from build123d import *

# Parameters (mm, degrees)
BOSS_EXTRUDE1_DEPTH = 6.35
SKETCH3_R           = 19.685
CUT_EXTRUDE1_DEPTH  = 7.35


with BuildPart() as part:
    # Sketch2 → Boss-Extrude1 (new body)
    with BuildSketch(Plane.XY):
        Polygon((0, 304.8), (0, 12.7), (127, 12.7), (127, 50.8), (254, 50.8), (254, 12.7), (431.8, 12.7), (431.8, 431.8), (215.9, 431.8), align=None)
    extrude(amount=BOSS_EXTRUDE1_DEPTH)

    # Sketch3 → Cut-Extrude1 (cut, through all)
    with BuildSketch(Plane.XY.offset(6.35)):
        with Locations((98.15, 150.3)):
            Circle(SKETCH3_R)
        with Locations((333.65, 150.3)):
            Circle(SKETCH3_R)
    extrude(amount=-CUT_EXTRUDE1_DEPTH, mode=Mode.SUBTRACT)


solid = part.part
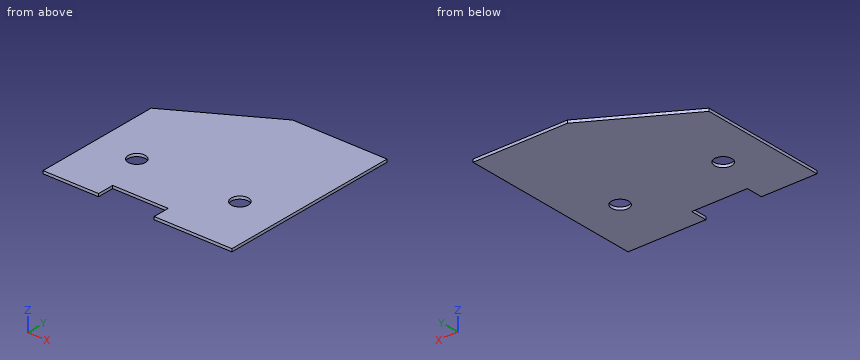
Verification items for the finished model (mm, model axes). Round coordinates to 2 decimals unless told otherwise and drop trailing zeros. Order: outer loops, then holes, each group sorted by start corner. A loop starts at its lowest first (then second) coordinate and runs counter-clockwise, first axis right, second up.
1. Section check D-D on x = 98.15. Record the cut outline in (y, z) (3 decimals).
Final values:
outline: (12.7, 0) - (130.615, 0) - (130.615, 6.35) - (12.7, 6.35) - close; (169.985, 0) - (362.535, 0) - (362.535, 6.35) - (169.985, 6.35) - close
2. Section check A-A on y = 150.3. Record the cut outline in (x, z) (3 decimals), then the cut area to 3 significant figures.
Final values:
outline: (0, 0) - (78.465, 0) - (78.465, 6.35) - (0, 6.35) - close; (117.835, 0) - (313.965, 0) - (313.965, 6.35) - (117.835, 6.35) - close; (353.335, 0) - (431.8, 0) - (431.8, 6.35) - (353.335, 6.35) - close
area: 2,240 mm2
3. Thickness scan on L1, parallel to X at y = 30, z = 6.25; L2, parallel to Y at x = 333.65, z = 3.5 (3 decimals); L3, parallel to Y at x = 238.5, z = 5. Record the ranges inside material, lowest first.
Final values:
L1: x = 0 to 127, 254 to 431.8
L2: y = 12.7 to 130.615, 169.985 to 431.8
L3: y = 50.8 to 431.8
4. Section check B-B on x = 333.65. Record the cut outline in (y, z) (3 decimals), then the cut area to 3 significant figures.
Final values:
outline: (12.7, 0) - (130.615, 0) - (130.615, 6.35) - (12.7, 6.35) - close; (169.985, 0) - (431.8, 0) - (431.8, 6.35) - (169.985, 6.35) - close
area: 2,410 mm2
5. Section check C-C on z = 1.5. Record the cut outline in (x, y) (3 decimals), then the cut area to 3 significant figures.
Final values:
outline: (0, 12.7) - (127, 12.7) - (127, 50.8) - (254, 50.8) - (254, 12.7) - (431.8, 12.7) - (431.8, 431.8) - (215.9, 431.8) - (0, 304.8) - close; hole circle Ø39.37 at (98.15, 150.3); hole circle Ø39.37 at (333.65, 150.3)
area: 160,000 mm2
